For this review, take the finished solid that the model builds, in its own axes (mm). Give positions to 0.01 mm unless a question says otherwise; leave off trailing zeros. Loops run counter-clockwise (first coordinate to the right, second up) from the corner with the lowest first, then second, coordinate; pieces in that order, holes last. Notation, with made-up numbers: (54, -3.5) - (95, -3.5) arc R20 ccw to (95, 33.5) - close; hole circle Ø2 at (51.5, -28.75). An arc over 180 degrees is marked (long way). Put each result on its own line as item: value.
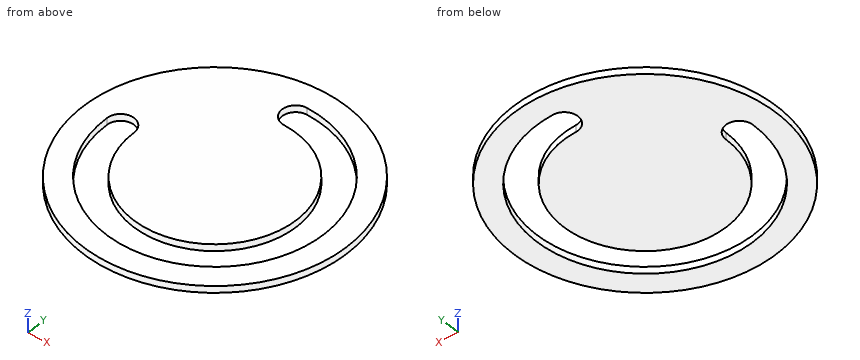
from build123d import *

# Parameters (mm, degrees)
SKETCH_1_R          = 9.7
EXTRUDE_1_DEPTH     = 0.5
CUT_EXTRUDE_1_DEPTH = 14.726980731


with BuildPart() as part:
    # 草图1 → 凸台-拉伸1 (new body)
    with BuildSketch(Plane.XY):
        Circle(SKETCH_1_R)
    extrude(amount=EXTRUDE_1_DEPTH)

    # 草图3 → 切除-拉伸1 (cut, through all)
    with BuildSketch(Plane.XY.offset(0.5)):
        with BuildLine():
            ThreePointArc((-8, 0), (5.656854249, -5.656854249), (0, 8))
            ThreePointArc((0, 8), (-1, 7), (0, 6))
            ThreePointArc((0, 6), (4.242640687, -4.242640687), (-6, 0))
            ThreePointArc((-6, 0), (-7, 1), (-8, 0))
        make_face()
    extrude(amount=-CUT_EXTRUDE_1_DEPTH, mode=Mode.SUBTRACT)


solid = part.part
1) Take a section at B-B on x = -3.5. State the section outline as (y, z) points.
Geometry check:
outline: (-9.05, 0) - (-7.19, 0) - (-7.19, 0.5) - (-9.05, 0.5) - close; (-4.87, 0) - (9.05, 0) - (9.05, 0.5) - (-4.87, 0.5) - close
2) Take a section at C-C on y = -2.5. State the section outline as (x, z) points, and give its area (3 significant figures).
Geometry check:
outline: (-9.37, 0) - (-7.6, 0) - (-7.6, 0.5) - (-9.37, 0.5) - close; (-5.45, 0) - (5.45, 0) - (5.45, 0.5) - (-5.45, 0.5) - close; (7.6, 0) - (9.37, 0) - (9.37, 0.5) - (7.6, 0.5) - close
area: 7.23 mm²
3) Take a section at A-A on y = 1.25. State the section outline as (x, z) points, and give its area (3 significant figures).
Geometry check:
outline: (-9.62, 0) - (5.87, 0) - (5.87, 0.5) - (-9.62, 0.5) - close; (7.9, 0) - (9.62, 0) - (9.62, 0.5) - (7.9, 0.5) - close
area: 8.60 mm²
4) Take a section at D-D on z = 0.1. State the section outline as (x, y) points, and give its area (3 significant figures).
Geometry check:
outline: circle Ø19.4 at (0, 0); hole (-8, 0) arc R8 ccw (long way) to (0, 8) arc R1 ccw to (0, 6) arc R6 cw (long way) to (-6, 0) arc R1 ccw to start
area: 226 mm²
5) Wall thickness on line 1 (Y direction, x = 1.75, z = 0.4); line 2 (X direction, y = -3.5, z = 0.45): over which ranges is each line inside the solid? List them lowest first.
Geometry check:
line 1: y = -9.54 to -7.81, -5.74 to 5.74, 7.81 to 9.54
line 2: x = -9.05 to -7.19, -4.87 to 4.87, 7.19 to 9.05
